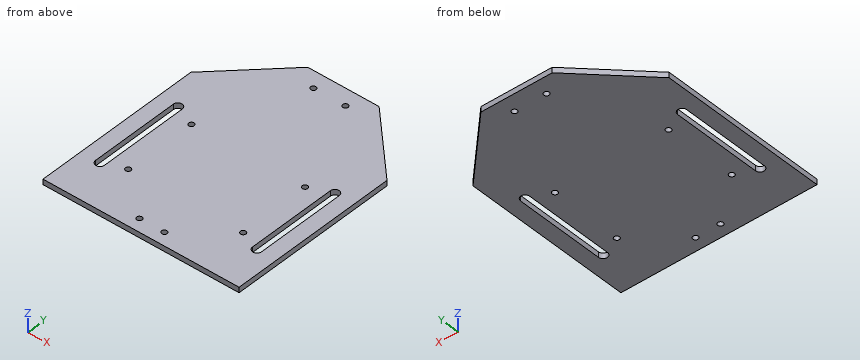
```python
from build123d import *

# Parameters (mm, degrees)
F0_W      = 55
F0_H      = 130
F1_DEPTH  = 3
F2_SIZE   = 35
F4_DEPTH  = 34.03176
F6_D      = 3
F8_D      = 3
F9_R      = 1.5
F10_DEPTH = 25
F11_R     = 1.5
F12_DEPTH = 25


with BuildPart() as f1:
    # F0 (on Top) → F1 (new body)
    with BuildSketch(Plane.XY):
        with Locations((27.5, 65)):
            Rectangle(F0_W, F0_H)
    extrude(amount=F1_DEPTH)

    # F2
    f2_edges = [f1.edges().sort_by_distance(p)[0] for p in [
        (55, 130, 1.5),
    ]]
    chamfer(f2_edges, length=F2_SIZE)

    # F3 (on face) → F4 (cut)
    with BuildSketch(Plane.XY.offset(3)):
        with BuildLine():
            ThreePointArc((46.534898, 74.060881), (44.034898, 76.560881), (41.534898, 74.060881))
            Line((41.534898, 74.060881), (41.534898, 24.060881))
            ThreePointArc((41.534898, 24.060881), (44.034898, 21.560881), (46.534898, 24.060881))
            Line((46.534898, 24.060881), (46.534898, 74.060881))
        make_face()
    extrude(amount=-F4_DEPTH, mode=Mode.SUBTRACT)

    # F6 (through all)
    with Locations(Plane.XY.offset(3)):
        with Locations((31.894885, 68.837039)):
            Hole(F6_D / 2)

    # F8 (through all)
    with Locations(Plane.XY.offset(3)):
        with Locations((32.258615, 28.699279)):
            Hole(F8_D / 2)

    # F9 (on face) → F10 (cut)
    with BuildSketch(Plane(origin=(0, 0, 0), x_dir=(1, 0, 0), z_dir=(0, 0, -1))):
        with Locations((7, -7)):
            Circle(F9_R)
    extrude(amount=-F10_DEPTH, mode=Mode.SUBTRACT)

    # F11 (on face) → F12 (cut)
    with BuildSketch(Plane.XY.offset(3)):
        with Locations((9, 121)):
            Circle(F11_R)
    extrude(amount=-F12_DEPTH, mode=Mode.SUBTRACT)

    # F14: F1 across plane


with BuildPart() as f1_1:
    add(f1.part)
    add(f1.part.mirror(Plane.YZ))


solid = f1_1.part
```
Model file for the job. Use its own axes, mm. Round coordinates to 2 decimals unless told otherwise and drop trailing zeros. Write each loop counter-clockwise with the first axis right and the second up, starting at its lowest first coordinate (ties: lowest second). Pieces come first, ordered by that corner, then holes. Notation, with made-up numbers: M 42,49 L 79,49 A29 cw 79,69 Z; hole C 4.5,14.5 d5. An arc over 180 degrees is marked long. Put each result on its own line as item: value.
Item 1: Cut at B-B (x = 45). List the corners of the cut face in (y, z).
Responses:
outline: M 0,0 L 21.75,0 L 21.75,3 L 0,3 Z; M 76.37,0 L 105,0 L 105,3 L 76.37,3 Z
Item 2: Cut at A-A (y = 7). List the corners of the cut face in (x, z), and give its area (3 significant figures).
Responses:
outline: M -55,0 L -8.5,0 L -8.5,3 L -55,3 Z; M -5.5,0 L 5.5,0 L 5.5,3 L -5.5,3 Z; M 8.5,0 L 55,0 L 55,3 L 8.5,3 Z
area: 312 mm²
Item 3: Flat gauge pins, fed straight in: P1, Ø3.5, axis at x = 7, y = 7, coming from the +Z side; P2, Ø2.5, axis at x = 32.26, y = 28.7, coming from the +Z side. Where does each tip first touch, or does it go through?
Responses:
P1: z = 3
P2: through
Item 4: Cut at D-D (z = 2.1). State how many separate pieces and enclosed holes the cut face has, and give its area (3 significant figures).
Responses:
separate pieces: 1
enclosed holes: 10
area: 12,500 mm²
Item 5: Cut at C-C (y = 121). List the corners of the cut face in (x, z), and give its area (3 significant figures).
Responses:
outline: M -29,0 L -10.5,0 L -10.5,3 L -29,3 Z; M -7.5,0 L 7.5,0 L 7.5,3 L -7.5,3 Z; M 10.5,0 L 29,0 L 29,3 L 10.5,3 Z
area: 156 mm²
Item 6: Probe L1, parallel to X at y = 39.5, z = 1.85; L2, parallel to X at y = 121, z = 0.9; L3, parallel to Y at x = 31.5, z = 0.65. List the from-to ranges inside material, lowest first. Write a range as from..to.
Responses:
L1: -55..-46.53, -41.53..41.53, 46.53..55
L2: -29..-10.5, -7.5..7.5, 10.5..29
L3: 0..27.41, 29.99..67.39, 70.28..118.5
